The listing builds one solid part. Answer for the finished solid, in the listing's coordinates (mm). A direction names the side the tool comes from. Coordinates: 2 decimals unless noted, no trailing zeros. Order: outer loops, then holes, each group sorted by start corner. A loop starts at its lowest first (then second) coordinate and runs counter-clockwise, first axis right, second up. Notation, with made-up numbers: (89.5, 13) -> (95.5, 13) arc R14 cw to (95.5, 37) -> close; hole circle Ø11 at (69, 70). An arc over 180 degrees is marked (long way). One line per question, with ' | ' between items.
Autodesk Inventor part; units mm, degrees
ref_plane "YZ Plane" through (0, 0, 0) normal (1, 0, 0) x (0, 1, 0)
ref_plane "XZ Plane" through (0, 0, 0) normal (0, 1, 0) x (-1, 0, 0)
ref_plane "XY Plane" through (0, 0, 0) normal (0, 0, 1) x (1, 0, 0)
sketch "スケッチ1" plane through (0, 0, 0) normal (0, 0, 1) x (1, 0, 0)
  circle A0 centre (0, 0) radius 2
  dimension "d0" = 4
extrude "押し出し1" add sketch "スケッチ1" along normal blind 30
sketch "スケッチ2" plane through (0, 0, 0) normal (0, 0, -1) x (-1, 0, 0)
  circle A0 centre (0, 0) radius 4
  dimension "d3" = 8
extrude "押し出し2" add sketch "スケッチ2" along normal blind 2.3
chamfer "面取り1" distance 2 angle 45 1 edges at (4, 0, 0)
thread "ねじ1"
sketch "スケッチ3" plane through (0, 0, -2.3) normal (0, 0, -1) x (-1, 0, 0)
  line L0 (1.7321, 0) -> (0.866, -1.5)
  line L1 (0.866, -1.5) -> (-0.866, -1.5)
  line L2 (-0.866, -1.5) -> (-1.7321, 0)
  line L3 (-1.7321, 0) -> (-0.866, 1.5)
  line L4 (-0.866, 1.5) -> (0.866, 1.5)
  line L5 (0.866, 1.5) -> (1.7321, 0)
  point P0 (0, 0)
  point P1 (0, 0)
  dimension "d11" = 3
extrude "押し出し3" cut sketch "スケッチ3" against normal blind 2
properties part number "M4皿ネジ　30" material "鉄 灰色"
Item 1: Each of these flat-tipped pins is pushed along its axis until it touches: pin 1 Ø1.4 at (x, z) = (-0.5, -1) entering from -Y; pin 2 Ø3.5 at (x, y) = (0.5, 0) entering from -Z; pin 3 Ø0.9 at (x, z) = (0.5, -1) entering from +Y. Where does it stop, or does it pass through?
Computed values:
pin 1: stops at y = -3.67 | pin 2: stops at z = -2.3 | pin 3: stops at y = 3.42
Item 2: Find the intervals of material crossed by L1, parallel to X at y = -1, z = 12; L2, parallel to X at y = 0.5, z = 28, in increasing order.
Computed values:
L1: x = -1.73 to 1.73 | L2: x = -1.94 to 1.94
Item 3: Determine the mould class of faces 1 (the face through (-2, 0, -2.3)), 2 (the face through (-1.293, 0.76, -1.314)), 3 (the face through (0.46, -2.08, -0.13)) for opening direction X: pulls with the +X half, pulls with the -X half, needs draft (parallel to the pull), parting line crosses it, or undercut.
Computed values:
face 1: needs draft | face 2: undercut | face 3: parting line crosses it
Item 4: Section B-B, the plane z = 12.5 is taken. Give the vertices of the cut face in (x, y).
Computed values:
outline: circle Ø4 at (0, 0)
Item 5: For faces 4 (the face through (0, 0, -0.3)), 5 (the face through (0, 2, 15)), 6 (the face through (0, 0, 30)), determine the directions among +Z, -Z, +X, -X, +Y, -Y from which every point of the face is accessible in a straight line to the end or side of a thin tool.
Computed values:
face 4: -Z | face 5: +Z | face 6: +Z, +X, -X, +Y, -Y
